```python
from build123d import *

# Parameters (mm, degrees)
EXTRUDE_2_DEPTH = 20
SCALE_1_SCALE   = 0.5


with BuildPart() as part:
    # 草图1 → 凸台-拉伸2 (new body)
    with BuildSketch(Plane.XY):
        with BuildLine():
            Line((-25, -30), (-25, 0))
            Line((-25, 0), (-210, 0))
            ThreePointArc((-210, 0), (0, -210), (210, 0))
            Line((210, 0), (25, 0))
            Line((25, 0), (25, -30))
            Line((25, -30), (0, -30))
            Line((0, -30), (-25, -30))
        make_face()
    extrude(amount=EXTRUDE_2_DEPTH)


with BuildPart() as part_1:
    # 缩放比例1: scaled about (0, -90.767415576, 10)
    add(part.part.scale(SCALE_1_SCALE).moved(Location((0, -45.383707788, 5))))


solid = part_1.part
```
Geometry: final body of the model. Coordinates: model frame, mm. A direction names the side the tool comes from. Give positions to 0.01 mm unless a question says otherwise; leave off trailing zeros. Write each loop counter-clockwise with the first axis right and the second up, starting at its lowest first coordinate (ties: lowest second). Pieces come first, ordered by that corner, then holes.
1. Section query B-B, the plane x = 48. Return loops of the section in (y, z).
2. Draft query along X for faces 3 (the cylindrical face through (-2.31, -150.36, 9.93)), 4 (the flat face through (-58, -45.384, 10)), 5 (the flat face through (0, -60.384, 10)). Return one class per face: released by +X, released by -X, zero draft, split by the parting line, or undercut.
3. Pin query (flat end, axial travel): P1, Ø5, axis at y = -102.5, z = 8.5, coming from the +X side; P2, Ø2, axis at x = -42, z = 11, coming from the -Y side; P3, Ø5, axis at x = -4.5, z = 11, coming from the +Y side. Return the tip coordinate at first contact, or that it passes through.
4. Reachability of faces 1 (the flat face through (-1, -85, 15)), 2 (the flat face through (-12.5, -53, 10)) from +Z, -Z, +X, -X, +Y, -Y: full face, straight path, thin tool, end or side. Return the list, or none.
5. Line query: probe 1 along X at (y, z) = (-56.5, 7.75); probe 2 along X at (y, z) = (-60, 9.5); probe 3 along Y at (x, z) = (1, 11). Output: solid intervals per line, ascending.
6. Section query C-C, the plane y = -90.5. Return loops of the section in (x, z), then the cut area to 3 significant figures.
7. Section query A-A, the plane z = 12.5. Return loops of the section in (x, y), then the cut area to 3 significant figures.
Computed:
1. outline: (-138.77, 5) - (-45.38, 5) - (-45.38, 15) - (-138.77, 15) - close
2. face 3: split by the parting line
2. face 4: zero draft
2. face 5: undercut
3. P1: stops at x = 89.68
3. P2: stops at y = -142.05
3. P3: stops at y = -60.38
4. face 1: +Z, +X, -X, +Y, -Y
4. face 2: +Z, -Z, +Y
5. probe 1: x = -104.41 to -12.5, 12.5 to 104.41
5. probe 2: x = -103.98 to -12.5, 12.5 to 103.98
5. probe 3: y = -150.38 to -60.38
6. outline: (-94.81, 5) - (94.81, 5) - (94.81, 15) - (-94.81, 15) - close
6. area: 1,900 mm2
7. outline: (-105, -45.38) arc R105 ccw to (105, -45.38) - (12.5, -45.38) - (12.5, -60.38) - (-12.5, -60.38) - (-12.5, -45.38) - close
7. area: 16,900 mm2
